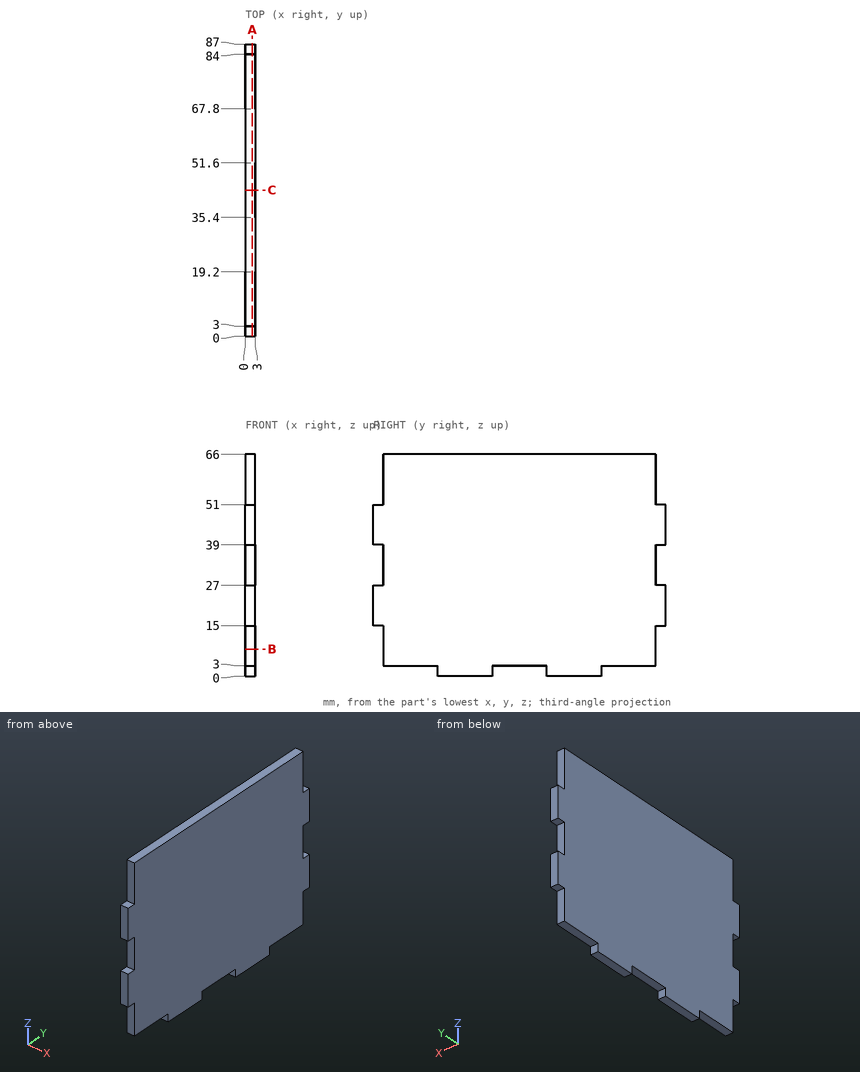
Could you check a few things on this drawing? It's one solid part, dimensions in mm from its lowest x, y, z. Give positions to 0.01 mm unless a question says otherwise; leave off trailing zeros. Order: outer loops, then holes, each group sorted by start corner. A loop starts at its lowest first (then second) coordinate and runs counter-clockwise, first axis right, second up. Notation, with made-up numbers: (6.5, 52) -> (10.5, 52) arc R7 cw to (10.5, 63) -> close; hole circle Ø10 at (63.25, 25.25). An arc over 180 degrees is marked (long way). Answer in a Markdown table with one row per item. Add a question column.
Item 1: Please list where these lines run through material, in increasing order: probe 1 along Z at (x, y) = (2.75, 38); probe 2 along Y at (x, z) = (0.25, 60.5).
Item 2: Imagine slicing it at A-A (x = 2.1). List the corners of the cut face in (y, z) for me.
Item 3: Imagine slicing it at C-C (y = 43.5). List the corners of the cut face in (x, z) for me.
Item 4: Imagine slicing it at B-B (z = 8). List the corners of the cut face in (x, y) for me, and give its area (3 significant figures).
Item 5: I'm going to push flat-ended pins straight in: P1, Ø0.9, axis at x = 1, z = 33, coming from the -Y side; P2, Ø0.9, axis at x = 1, y = 8.5, coming from the -Z side; P3, Ø0.9, axis at x = 1.5, y = 85, coming from the +Z side. Where does each tip first touch, or does it pass through?
Result:
| question | item | result |
|---|---|---|
| 1 | probe 1 | 3 to 66 |
| 1 | probe 2 | 3 to 84 |
| 2 | outline | (0, 15) -> (3, 15) -> (3, 3) -> (19.2, 3) -> (19.2, 0) -> (35.4, 0) -> (35.4, 3) -> (51.6, 3) -> (51.6, 0) -> (67.8, 0) -> (67.8, 3) -> (84, 3) -> (84, 15) -> (87, 15) -> (87, 27) -> (84, 27) -> (84, 39) -> (87, 39) -> (87, 51) -> (84, 51) -> (84, 66) -> (3, 66) -> (3, 51) -> (0, 51) -> (0, 39) -> (3, 39) -> (3, 27) -> (0, 27) -> close |
| 3 | outline | (0, 3) -> (3, 3) -> (3, 66) -> (0, 66) -> close |
| 4 | outline | (0, 3) -> (3, 3) -> (3, 84) -> (0, 84) -> close |
| 4 | area | 243 mm2 |
| 5 | P1 | y = 3 |
| 5 | P2 | z = 3 |
| 5 | P3 | z = 51 |
